Can you work these out from the model? Positions are in its coordinate system, mm. Round coordinates to 2 decimals unless told otherwise and drop trailing zeros. Loops run counter-clockwise (first coordinate to the right, second up) from the corner with the lowest first, then second, coordinate; pieces in that order, holes last. Notation, with made-up numbers: M 42.25,-29.75 L 50.25,-29.75 A20 ccw 50.25,-2.75 Z; hole C 71.5,26 d3. An arc over 180 degrees is marked long. Return JSON: item names as keys, results as strings.
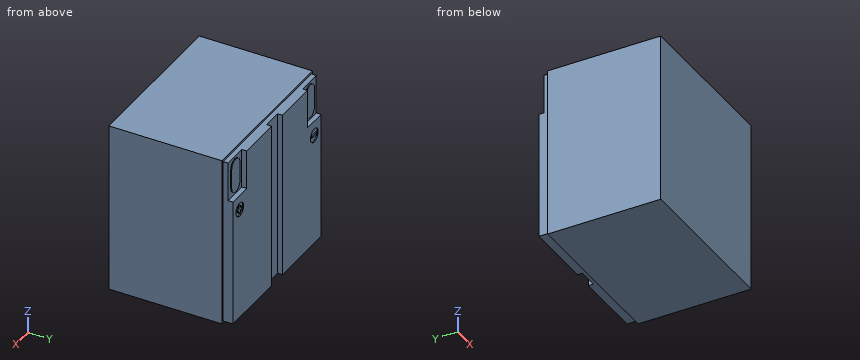
```python
from build123d import *

# Parameters (mm, degrees)
SKETCH1_R           = 7
SKETCH1_W           = 8
SKETCH1_H           = 2
SKETCH1_W_2         = 2
SKETCH1_H_2         = 8
BOSS_EXTRUDE3_DEPTH = 125
SKETCH1_6_R         = 7
BOSS_EXTRUDE4_DEPTH = 124
SKETCH1_7_W         = 25
SKETCH1_7_H         = 40
SKETCH1_7_W_2       = 20
SKETCH1_7_H_2       = 170
BOSS_EXTRUDE5_DEPTH = 120
BOSS_EXTRUDE6_DEPTH = 121
SKETCH1_10_W        = 165
SKETCH1_10_H        = 174
BOSS_EXTRUDE7_DEPTH = 115


with BuildPart() as part:
    # Sketch1 → Boss-Extrude3 (new body)
    # profile 1 of 5: a face of its own
    with BuildSketch(Plane(origin=(0, 0, 0), x_dir=(1, 0, 0), z_dir=(0, 1, 0))):
        Polygon((80.5, -45), (80.5, 85), (10, 85), (10, -85), (55.5, -85), (55.5, -45), align=None)
        with Locations(Location((68, -30, 0), (0, 0, 270))):
            Circle(SKETCH1_R, mode=Mode.SUBTRACT)
    # profile 2 of 5: a face of its own
    with BuildSketch(Plane(origin=(0, 0, 0), x_dir=(1, 0, 0), z_dir=(0, 1, 0))):
        Polygon((-10, -85), (-10, 85), (-80.5, 85), (-80.5, -45), (-55.5, -45), (-55.5, -85), align=None)
        with Locations(Location((-68, -30, 0), (0, 0, 270))):
            Circle(SKETCH1_R, mode=Mode.SUBTRACT)
    # profile 3 of 5: a face of its own
    with BuildSketch(Plane(origin=(0, 0, 0), x_dir=(1, 0, 0), z_dir=(0, 1, 0))):
        with Locations((-68, -30)):
            Rectangle(SKETCH1_W, SKETCH1_H)
    # profile 4 of 5: a face of its own
    with BuildSketch(Plane(origin=(0, 0, 0), x_dir=(1, 0, 0), z_dir=(0, 1, 0))):
        with Locations((68, -30)):
            Rectangle(SKETCH1_W_2, SKETCH1_H_2)
    # profile 5 of 5: a face of its own
    with BuildSketch(Plane(origin=(0, 0, 0), x_dir=(1, 0, 0), z_dir=(0, 1, 0))):
        with Locations((68, -30)):
            Rectangle(SKETCH1_W, SKETCH1_H)
    extrude(amount=BOSS_EXTRUDE3_DEPTH)

    # Sketch1_6 → Boss-Extrude4 (add)
    with BuildSketch(Plane(origin=(0, 0, 0), x_dir=(1, 0, 0), z_dir=(0, 1, 0))):
        with Locations(Location((-68, -30, 0), (0, 0, 270))):
            Circle(SKETCH1_6_R)
        with Locations(Location((68, -30, 0), (0, 0, 90))):
            Circle(SKETCH1_6_R)
    extrude(amount=BOSS_EXTRUDE4_DEPTH)

    # Sketch1_7 → Boss-Extrude5 (add)
    # profile 1 of 3: a face of its own
    with BuildSketch(Plane(origin=(0, 0, 0), x_dir=(1, 0, 0), z_dir=(0, 1, 0))):
        with Locations((-68, -65)):
            Rectangle(SKETCH1_7_W, SKETCH1_7_H)
        with BuildLine():
            ThreePointArc((-75.5, -55), (-68, -47.5), (-60.5, -55))
            Line((-60.5, -55), (-60.5, -75))
            ThreePointArc((-60.5, -75), (-68, -82.5), (-75.5, -75))
            Line((-75.5, -75), (-75.5, -55))
        make_face(mode=Mode.SUBTRACT)
    # profile 2 of 3: a face of its own
    with BuildSketch(Plane(origin=(0, 0, 0), x_dir=(1, 0, 0), z_dir=(0, 1, 0))):
        with Locations((68, -65)):
            Rectangle(SKETCH1_7_W, SKETCH1_7_H)
        with BuildLine():
            Line((60.5, -75), (60.5, -55))
            ThreePointArc((60.5, -55), (68, -47.5), (75.5, -55))
            Line((75.5, -55), (75.5, -75))
            ThreePointArc((75.5, -75), (68, -82.5), (60.5, -75))
        make_face(mode=Mode.SUBTRACT)
    # profile 3 of 3: a face of its own
    with BuildSketch(Plane(origin=(0, 0, 0), x_dir=(1, 0, 0), z_dir=(0, 1, 0))):
        Rectangle(SKETCH1_7_W_2, SKETCH1_7_H_2)
    extrude(amount=BOSS_EXTRUDE5_DEPTH)

    # Sketch1_8 → Boss-Extrude6 (add)
    with BuildSketch(Plane(origin=(0, 0, 0), x_dir=(1, 0, 0), z_dir=(0, 1, 0))):
        with BuildLine():
            ThreePointArc((75.5, -75), (68, -82.5), (60.5, -75))
            Line((60.5, -75), (60.5, -55))
            ThreePointArc((60.5, -55), (68, -47.5), (75.5, -55))
            Line((75.5, -55), (75.5, -75))
        make_face()
        with BuildLine():
            Line((-75.5, -55), (-75.5, -75))
            ThreePointArc((-75.5, -75), (-68, -82.5), (-60.5, -75))
            Line((-60.5, -75), (-60.5, -55))
            ThreePointArc((-60.5, -55), (-68, -47.5), (-75.5, -55))
        make_face()
    extrude(amount=BOSS_EXTRUDE6_DEPTH)

    # Sketch1_10 → Boss-Extrude7 (add)
    with BuildSketch(Plane(origin=(0, 0, 0), x_dir=(1, 0, 0), z_dir=(0, 1, 0))):
        Rectangle(SKETCH1_10_W, SKETCH1_10_H)
    extrude(amount=BOSS_EXTRUDE7_DEPTH)


solid = part.part
```
Q1. If I drill on line 1 along X through (y, z) = (124.6, 30); line 2 along Y through (x, z) = (61.5, 52.5), over which ranges is the centre line in solid material (lowest first)?
Results:
{"line 1": "x = -80.5 to -75, -72 to -64, -61 to -10, 10 to 61, 64 to 72, 75 to 80.5", "line 2": "y = 0 to 121"}
Q2. I'm going to push flat-ended pins straight in: pin 1 Ø6 at (x, z) = (-3.5, -10) entering from +Y; pin 2 Ø2.5 at (x, y) = (-64.5, 121.5) entering from +Z; pin 3 Ø1.1 at (x, y) = (68, 124.5) entering from -Z. Where does each tip first touch, or does it pass through?
Results:
{"pin 1": "stops at y = 120", "pin 2": "stops at z = 82.12", "pin 3": "stops at z = -85"}
Q3. Suppose I cut it at A-A, the plane x = 3.5. Please give me the cut outline in (y, z).
Results:
{"outline": "M 0,-87 L 115,-87 L 115,-85 L 120,-85 L 120,85 L 115,85 L 115,87 L 0,87 Z"}
